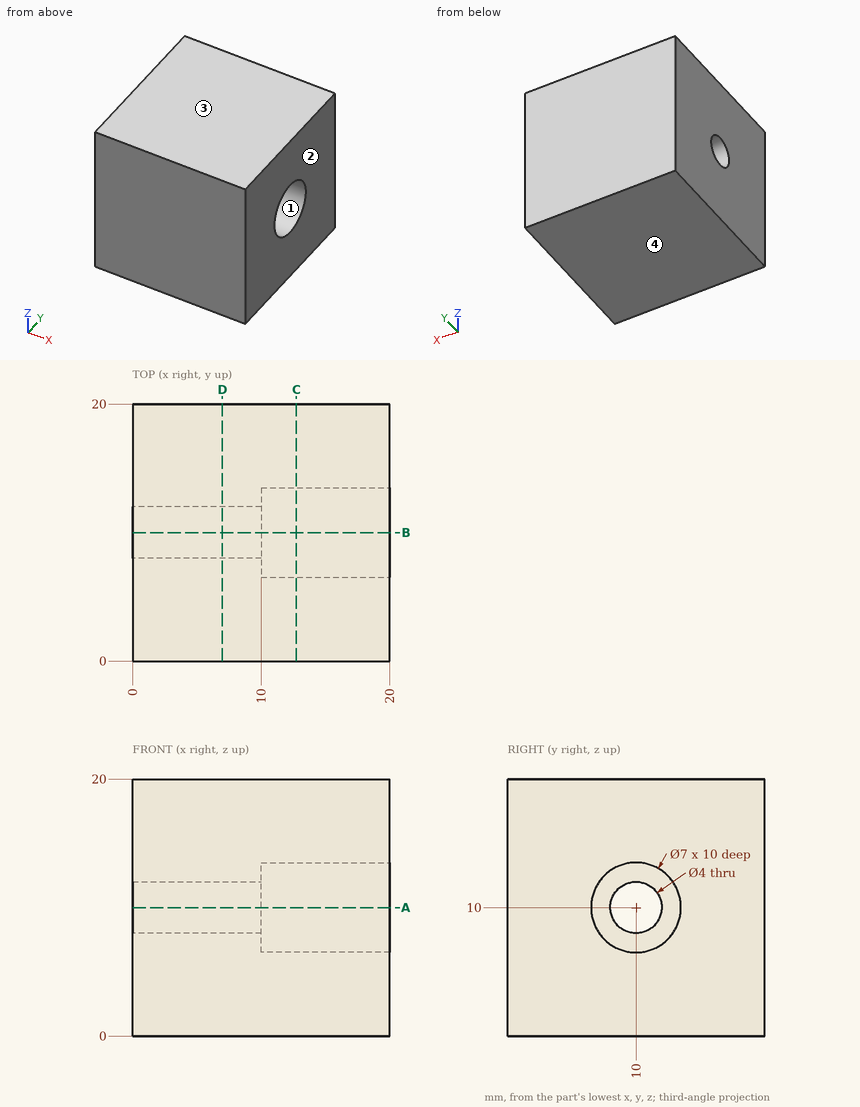
Verification items for this drawing (mm, ordinates from the low corner). Coordinates: 2 decimals unless noted, no trailing zeros. Order: outer loops, then holes, each group sorted by start corner. A loop starts at its lowest first (then second) coordinate and runs counter-clockwise, first axis right, second up. Notation, with made-up numbers: M 12.5,45.5 L 33.5,45.5 A13 cw 33.5,59.5 Z; hole C -8,10 d4. An arc over 180 degrees is marked long. Use CSV: the item, a comma, the result in double quotes.
Item 1: Cross-section at D-D on x = 7. Record the cut outline in (y, z).
Returned:
outline,"M 0,0 L 20,0 L 20,20 L 0,20 Z; hole C 10,10 d4"
Item 2: Cross-section at C-C on x = 12.75. Record the cut outline in (y, z).
Returned:
outline,"M 0,0 L 20,0 L 20,20 L 0,20 Z; hole C 10,10 d7"
Item 3: Mould release check, pull along Z, two halves, no side actions. Record for the marked faces 1, 2, 3 and 4: pulls with the +Z half, pulls with the -Z half, needs draft (parallel to the pull), parting line crosses it, or undercut.
Returned:
face 1,"undercut"
face 2,"needs draft"
face 3,"pulls with the +Z half"
face 4,"pulls with the -Z half"
Item 4: Thickness scan on line 1 along Y through (x, z) = (6.25, 10); line 2 along Y through (x, z) = (16.75, 10); line 3 along Z through (x, y) = (16.25, 11.5). Record the ranges inside material, lowest first.
Returned:
line 1,"y = 0 to 8, 12 to 20"
line 2,"y = 0 to 6.5, 13.5 to 20"
line 3,"z = 0 to 6.84, 13.16 to 20"
Item 5: Cross-section at A-A on z = 10. Record the cut outline in (x, y), then the cut area to 3 significant figures.
Returned:
outline,"M 0,0 L 20,0 L 20,6.5 L 10,6.5 L 10,8 L 0,8 Z; M 0,12 L 10,12 L 10,13.5 L 20,13.5 L 20,20 L 0,20 Z"
area,"290 mm2"
Item 6: Gauge pin test, flat end, axial feed: pin 1 Ø3.5 at (y, z) = (10.5, 10.5) entering from +X. Record the tip position at first contact, or that the pin passes through.
Returned:
pin 1,"stops at x = 10"
